from build123d import *

# Parameters (mm, degrees)
F0_W     = 58.1890903413
F0_H     = 43.9015906304
F1_DEPTH = 25.4
F2_R     = 6.0588899817
F3_DEPTH = 34.544
F4_W     = 46.7590875924
F4_H     = 32.9911382869
F5_DEPTH = 25.4
F6_R     = 7.896006859
F7_DEPTH = 53.086


with BuildPart() as f1:
    # F0 (on Front) → F1 (new body)
    with BuildSketch(Plane.XZ):
        with Locations((3.1172726303, -6.3644321635)):
            Rectangle(F0_W, F0_H)
    extrude(amount=F1_DEPTH)

    # F2 (on face) → F3 (join)
    with BuildSketch(Plane(origin=(-25.9772725403, 0, 0), x_dir=(0, -1, 0), z_dir=(-1, 0, 0))):
        with Locations((12.4690905213, -6.2345452607)):
            Circle(F2_R)
    extrude(amount=F3_DEPTH)

    # F4 (on face) → F5 (join)
    with BuildSketch(Plane(origin=(0, 0, 0), x_dir=(-1, 0, 0), z_dir=(0, 1, 0))):
        with Locations((-1.8184091896, -6.3644326292)):
            Rectangle(F4_W, F4_H)
    extrude(amount=F5_DEPTH)

    # F6 (on face) → F7 (join)
    with BuildSketch(Plane(origin=(0, 25.4, 0), x_dir=(-1, 0, 0), z_dir=(0, 1, 0))):
        with Locations((-2.8758263215, -6.9701997563)):
            Circle(F6_R)
    extrude(amount=F7_DEPTH)


solid = f1.part
Read the model definition and answer for the solid it produces. Units are mm, in the model's axes. A direction names the side the tool comes from. Give positions to 0.01 mm unless a question says otherwise; leave off trailing zeros. Write each loop counter-clockwise with the first axis right and the second up, starting at its lowest first coordinate (ties: lowest second). Pieces come first, ordered by that corner, then holes. Notation, with made-up numbers: (87, -0.5) -> (138, -0.5) arc R24 ccw to (138, 10.5) -> close; hole circle Ø7 at (55, 71.5). An arc over 180 degrees is marked (long way). Answer as a JSON object with one key per item and string values. Group by question number.
1) Find section B-B (x = 19). Write down the section's boundary in (y, z).
2) Find section C-C (y = 24). Write down the section's boundary in (x, z).
3) Find section D-D (x = -1.5). Write down the section's boundary in (y, z).
4) Consider L1, parallel to X at y = 3, z = -9.5; L2, parallel to X at y = 26, z = -7; L3, parallel to Y at x = 2, z = 3.5. Determine where each line is inside the solid, lowest interval first. Write a range as from..to.
5) Each of these flat-tipped pins is pushed along its axis until it touches: P1, Ø12.5, axis at y = 13.5, z = -10.5, coming from the -X side; P2, Ø4, axis at y = 26.5, z = -12, coming from the +X side; P3, Ø1, axis at x = 7.5, y = 42.5, coming from the -Z side. Where does it stop, or does it pass through?
6) Find section A-A (z = 7). Write down the section's boundary in (x, y), and give its area (3 significant figures).
7) A tool of negligible diameter and unlimited length cuts with its end or side. For faces 1 (the cylindrical face through (-43.007, -6.416, -5.968)), 2 (the flat face through (2, 13, 10.131)), 3 (the flat face through (-21.561, 13, -7)), 4 (the flat face through (25.198, 13, -7)), 5 (the cylindrical face through (-4.656, 51.571, -4.598)), from which of +Z, -Z, +X, -X, +Y, -Y can it reach the whole face along a straight path? Write none if from no direction.
Values follow:
{
 "1": {"outline": "(-25.4, -28.32) -> (0, -28.32) -> (0, -22.86) -> (25.4, -22.86) -> (25.4, 10.13) -> (0, 10.13) -> (0, 15.59) -> (-25.4, 15.59) -> close"},
 "2": {"outline": "(-21.56, -22.86) -> (25.2, -22.86) -> (25.2, 10.13) -> (-21.56, 10.13) -> close"},
 "3": {"outline": "(-25.4, -28.32) -> (0, -28.32) -> (0, -22.86) -> (25.4, -22.86) -> (25.4, -13.54) -> (78.49, -13.54) -> (78.49, -0.4) -> (25.4, -0.4) -> (25.4, 10.13) -> (0, 10.13) -> (0, 15.59) -> (-25.4, 15.59) -> close"},
 "4": {"L1": "x = -21.56..25.2", "L2": "x = -5.02..10.77", "L3": "y = -25.4..25.4"},
 "5": {"P1": "stops at x = -21.56", "P2": "stops at x = 25.2", "P3": "stops at z = -13.7"},
 "6": {"outline": "(-25.98, -25.4) -> (32.21, -25.4) -> (32.21, 0) -> (25.2, 0) -> (25.2, 25.4) -> (-21.56, 25.4) -> (-21.56, 0) -> (-25.98, 0) -> close", "area": "2,670 mm2"},
 "7": {"face 1": "-X", "face 2": "+Z, +X, -X, +Y", "face 3": "+Z, -Z, -X, +Y", "face 4": "+Z, -Z, +X, +Y", "face 5": "+Y"}
}
